Source: three-view drawing plus pictorial views. Frame: mm from the lowest corner of the part. A direction names the side the tool comes from. Give positions to 0.01 mm unless a question says otherwise; leave off trailing zeros. Loops run counter-clockwise (first coordinate to the right, second up) from the corner with the lowest first, then second, coordinate; pieces in that order, holes last. Notation, with made-up numbers: (67, 32.5) -> (74, 32.5) arc R16 cw to (74, 55.5) -> close; hole circle Ø3 at (46, -3.5). An arc over 180 degrees is marked (long way). Put each result on its own line as item: value.
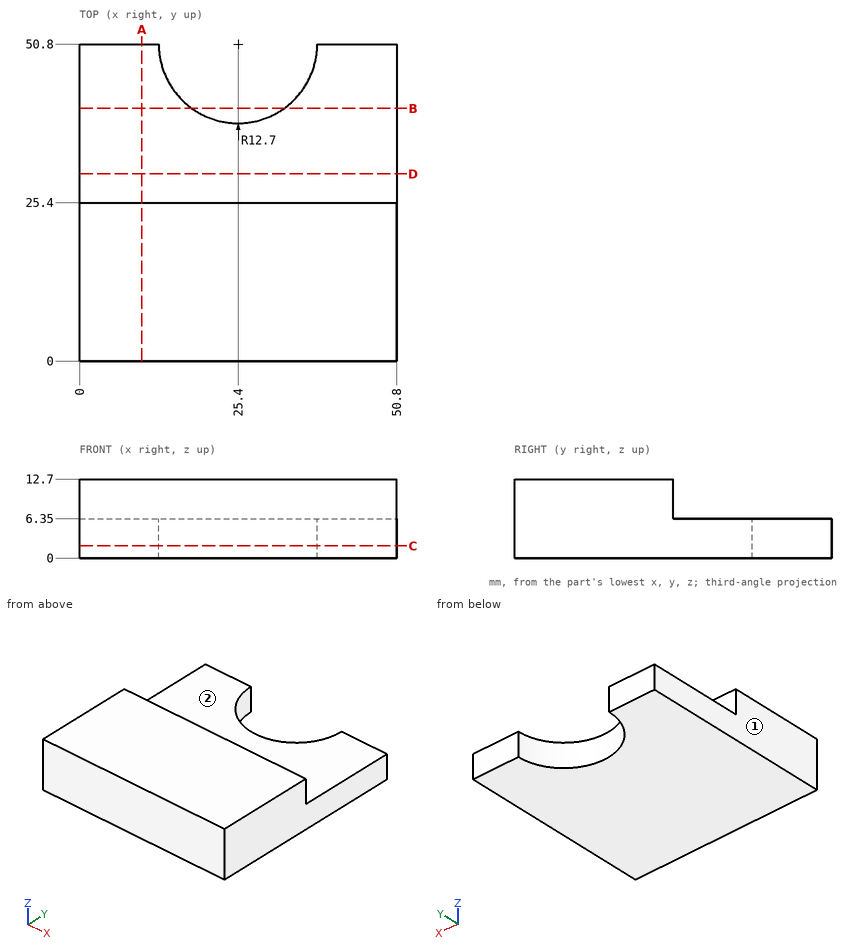
(1) Section C-C on z = 2. Return loops of the section in (x, y).
Calculated:
outline: (0, 0) -> (50.8, 0) -> (50.8, 50.8) -> (38.1, 50.8) arc R12.7 cw to (12.7, 50.8) -> (0, 50.8) -> close
(2) Line query: probe 1 along Z at (x, y) = (30, 37); probe 2 along Y at (x, z) = (48.5, 8.75); probe 3 along Y at (x, z) = (15, 1). Output: solid intervals per line, ascending. Write a range as from..to.
Calculated:
probe 1: z = 0..6.35
probe 2: y = 0..25.4
probe 3: y = 0..43.51
(3) Section A-A on x = 10. Return loops of the section in (y, z), then the cut area to 3 significant figures.
Calculated:
outline: (0, 0) -> (50.8, 0) -> (50.8, 6.35) -> (25.4, 6.35) -> (25.4, 12.7) -> (0, 12.7) -> close
area: 484 mm²
(4) Section B-B on y = 40.5. Return loops of the section in (x, z), then the cut area to 3 significant figures.
Calculated:
outline: (0, 0) -> (17.97, 0) -> (17.97, 6.35) -> (0, 6.35) -> close; (32.83, 0) -> (50.8, 0) -> (50.8, 6.35) -> (32.83, 6.35) -> close
area: 228 mm²
(5) First-contact query: P1, Ø12, axis at x = 33.5, y = 45.5, coming from the +Z side; P2, Ø3, axis at x = 19.5, z = 9.5, coming from the +Y side. Flat tips, straight axial feed; report the tip coordinate or a pass-through.
Calculated:
P1: stops at z = 6.35
P2: stops at y = 25.4
(6) Reachability of the marked faces 1 and 2 from +Z, -Z, +X, -X, +Y, -Y: full face, straight path, thin tool, end or side. Return the list, or none.
Calculated:
face 1: +Z, -Z, -X, +Y, -Y
face 2: +Z, +X, -X, +Y
(7) Section D-D on y = 30. Return loops of the section in (x, z), then the cut area to 3 significant figures.
Calculated:
outline: (0, 0) -> (50.8, 0) -> (50.8, 6.35) -> (0, 6.35) -> close
area: 323 mm²
